Model file for the job. Use its own axes, mm. A direction names the side the tool comes from. Round coordinates to 2 decimals unless told otherwise and drop trailing zeros. Loops run counter-clockwise (first coordinate to the right, second up) from the corner with the lowest first, then second, coordinate; pieces in that order, holes last. Notation, with made-up numbers: M -37,4 L 6,4 A35 cw 6,37 Z; hole C 25.25,58 d1. An arc over 180 degrees is marked long. Answer in a Markdown table with one row per item.
from build123d import *

# Parameters (mm, degrees)
SKETCH_W        = 28
SKETCH_H        = 6
SKETCH_R        = 1.6
PAD_DEPTH       = 5
POCKET_DEPTH    = 5.001
SKETCH007_R     = 1.6
POCKET001_DEPTH = 6.001


with BuildPart() as part:
    # Sketch → Pad (new body, symmetric)
    with BuildSketch(Plane.YZ):
        with Locations((0, 3)):
            Rectangle(SKETCH_W, SKETCH_H)
        with Locations((0, 2.8)):
            Circle(SKETCH_R, mode=Mode.SUBTRACT)
    extrude(amount=PAD_DEPTH, both=True)

    # Sketch006 → Pocket (cut, through all)
    with BuildSketch(Plane.YZ):
        Polygon((1.616581, 0), (3.233162, 2.8), (1.616581, 5.6), (-1.616581, 5.6), (-3.233162, 2.8), (-1.616581, 0), align=None)
    extrude(amount=-POCKET_DEPTH, mode=Mode.SUBTRACT)

    # Sketch007 → Pocket001 (cut, through all)
    with BuildSketch(Plane.XY):
        with Locations((0, 10)):
            Circle(SKETCH007_R)
        with Locations((0, -10)):
            Circle(SKETCH007_R)
    extrude(amount=POCKET001_DEPTH, mode=Mode.SUBTRACT)


with BuildPart() as part_1:
    # Body002 placement: moved
    add(part.part.moved(Location((0, 0, 8))))


solid = part_1.part
1. Mould opens along Y. For faces 4 (the flat face through (-2.465, 2.414, 9.38)), 5 (the flat face through (0, 14, 11)), 6 (the flat face through (5, 0, 9)) say: +Y half, -Y half, draft (parallel to the pull), parting line (faces both ways), or undercut.
Verdict:
| item | result |
|---|---|
| face 4 | undercut |
| face 5 | +Y half |
| face 6 | draft |
2. Saw through at C-C (z = 11.5). Write the cut outline in (x, y).
Verdict:
| item | result |
|---|---|
| outline | M -5,-14 L 5,-14 L 5,-1.44 L 0,-1.44 L 0,-2.83 L -5,-2.83 Z; M -5,2.83 L 0,2.83 L 0,1.44 L 5,1.44 L 5,14 L -5,14 Z; hole C 0,-10 d3.2; hole C 0,10 d3.2 |
3. Saw through at D-D (x = 3). Write the cut outline in (y, z), and give its area (3 significant figures).
Verdict:
| item | result |
|---|---|
| outline | M -14,8 L 14,8 L 14,14 L -14,14 Z; hole C 0,10.8 d3.2 |
| area | 160 mm² |
4. Saw through at A-A (y = -10). Write the cut outline in (x, z).
Verdict:
| item | result |
|---|---|
| outline | M -5,8 L -1.6,8 L -1.6,14 L -5,14 Z; M 1.6,8 L 5,8 L 5,14 L 1.6,14 Z |
5. Wall check: probe 1 along Z at (x, y) = (2.5, 0); probe 2 along Y at (x, z) = (3.3, 10.8); probe 3 along X at (y, z) = (10, 10.5). Give the ranges that are in metal, low to high.
Verdict:
| item | result |
|---|---|
| probe 1 | z = 8 to 9.2, 12.4 to 14 |
| probe 2 | y = -14 to -1.6, 1.6 to 14 |
| probe 3 | x = -5 to -1.6, 1.6 to 5 |
6. Pin check, flat tip, straight feed: pin 1 (1 mm diameter, centred on x = -2, y = 0, fed in from -Z). Stop position of the tip, or through.
Verdict:
| item | result |
|---|---|
| pin 1 | stops at z = 13.6 |
7. Tool access for faces 1 (the flat face through (-2, 0, 13.6)), 2 (the cylindrical face through (2.46, 0.86, 12.15)), 3 (the flat face through (-2.465, -2.414, 12.22)): list every direction of +Z, -Z, +X, -X, +Y, -Y with a clear straight run to the whole face (end or side of a thin tool).
Verdict:
| item | result |
|---|---|
| face 1 | -Z, -X |
| face 2 | +X, -X |
| face 3 | -X |
8. Saw through at B-B (x = -2.5). Write the cut outline in (y, z).
Verdict:
| item | result |
|---|---|
| outline | M -14,8 L -1.62,8 L -3.23,10.8 L -1.62,13.6 L 1.62,13.6 L 3.23,10.8 L 1.62,8 L 14,8 L 14,14 L -14,14 Z |
